Could you check a few things on this drawing? It's one solid part, dimensions in mm from its lowest x, y, z. Round coordinates to 2 decimals unless told otherwise and drop trailing zeros. Order: outer loops, then holes, each group sorted by start corner. A loop starts at its lowest first (then second) coordinate and runs counter-clockwise, first axis right, second up.
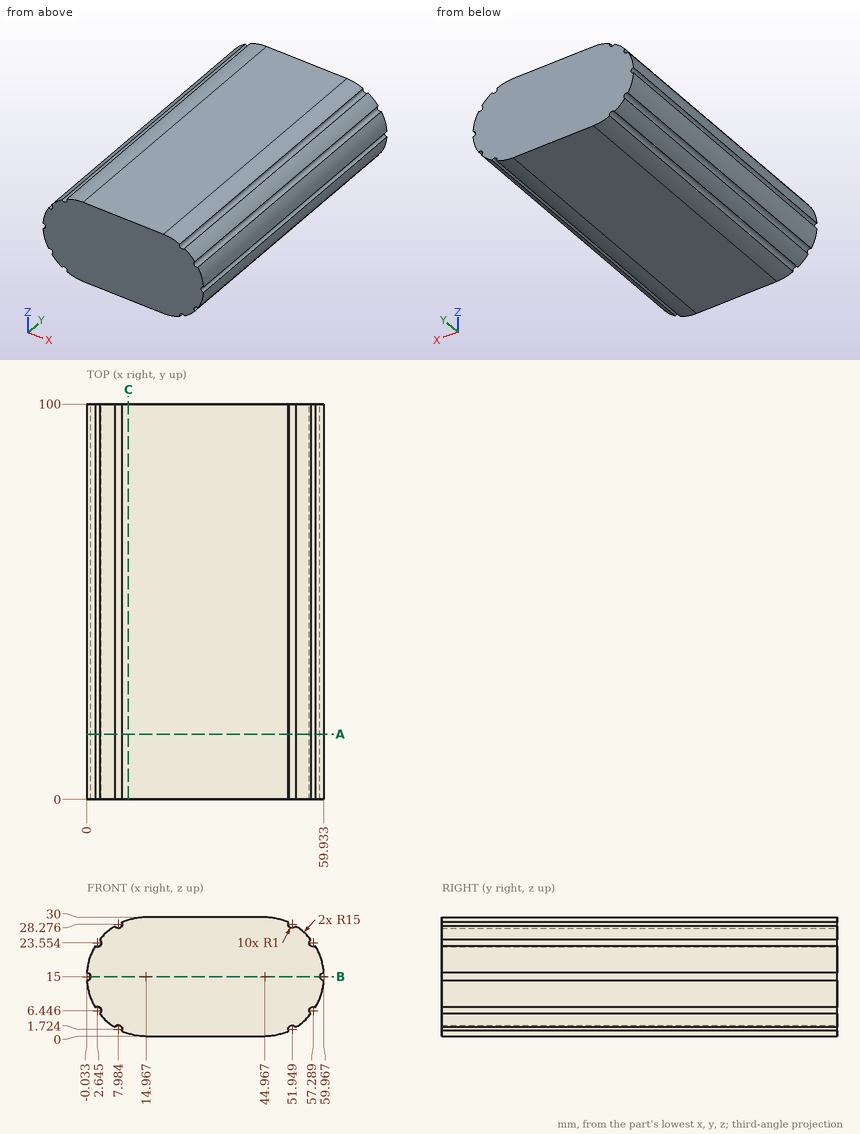
1) If we section it at B-B (z = 15): Write out the boundary of the cut face in (x, y), plus the area to 3 significant figures.
2) I need wall thicknesses on line 1 (Z direction, x = 56.5, y = 35.5); line 2 (Z direction, x = 47.5, y = 38.5) (1 decimal); line 3 (X direction, y = 11.5, z = 23.5). Which ranges of each line are inside material? Lowest first, please.
3) If we section it at A-A (y = 16.5): Write out the boundary of the cut face in (x, z) (1 decimal).
4) I'm going to push flat-ended pins straight in: pin 1 (8 mm diameter, centred on y = 68.5, z = 21, fed in from +X); pin 2 (1 mm diameter, centred on y = 19, z = 6, fed in from -X). Where does each tip first touch, or does it pass through?
5) If we section it at C-C (x = 10.5): Write out the boundary of the cut face in (y, z).
Solutions:
1. outline: (0.97, 0) - (58.97, 0) - (58.97, 100) - (0.97, 100) - close
1. area: 5,800 mm2
2. line 1: z = 5.41 to 5.83, 7.06 to 22.94, 24.17 to 24.59
2. line 2: z = 0.2 to 29.8
2. line 3: x = 3.64 to 56.29
3. outline: (0, 14) arc R15 ccw to (2.1, 7.3) arc R1 cw to (3.2, 5.6) arc R15 ccw to (7.1, 2.2) arc R1 cw to (8.9, 1.3) arc R15 ccw to (15, 0) - (45, 0) arc R15 ccw to (51, 1.3) arc R1 cw to (52.8, 2.2) arc R15 ccw to (56.7, 5.6) arc R1 cw to (57.8, 7.3) arc R15 ccw to (59.9, 14) arc R1 cw to (59.9, 16) arc R15 ccw to (57.8, 22.7) arc R1 cw to (56.7, 24.4) arc R15 ccw to (52.8, 27.8) arc R1 cw to (51, 28.7) arc R15 ccw to (45, 30) - (15, 30) arc R15 ccw to (8.9, 28.7) arc R1 cw to (7.1, 27.8) arc R15 ccw to (3.2, 24.4) arc R1 cw to (2.1, 22.7) arc R15 ccw to (0, 16) arc R1 cw to start
4. pin 1: stops at x = 59.83
4. pin 2: stops at x = 3.24
5. outline: (0, 0.68) - (100, 0.68) - (100, 29.32) - (0, 29.32) - close
